```python
from build123d import *

# Parameters (mm, degrees)
SKETCH1_R           = 17
SKETCH1_R_2         = 15
BOSS_EXTRUDE1_DEPTH = 10
BOSS_EXTRUDE2_START = -10
BOSS_EXTRUDE2_DEPTH = 10
CIRPATTERN1_COUNT   = 24


with BuildPart() as part:
    # Sketch1 → Boss-Extrude1 (new body)
    with BuildSketch(Plane.XY):
        Circle(SKETCH1_R)
        Circle(SKETCH1_R_2, mode=Mode.SUBTRACT)
    extrude(amount=BOSS_EXTRUDE1_DEPTH)

    # Sketch2 → Boss-Extrude2 (add)
    with BuildSketch(Plane.XY.offset(10).offset(BOSS_EXTRUDE2_START)):
        with BuildLine():
            ThreePointArc((-2.218945268, 16.854562643), (0, 17.5), (2.218945268, 16.854562643))
            ThreePointArc((2.218945268, 16.854562643), (0, 17), (-2.218945268, 16.854562643))
        make_face()
    boss_extrude2 = extrude(amount=BOSS_EXTRUDE2_DEPTH)

    # CirPattern1: Boss-Extrude2 ×24 about axis
    cirpattern1_axis = Axis((0, 0, 0), (0, 0, 1))
    for i in range(1, CIRPATTERN1_COUNT):
        add(boss_extrude2.rotate(cirpattern1_axis, i * 360 / CIRPATTERN1_COUNT))


solid = part.part
```
Could you check a few things on this model? Use its own coordinates, in mm. Round coordinates to 2 decimals unless told otherwise and drop trailing zeros. Loops run counter-clockwise (first coordinate to the right, second up) from the corner with the lowest first, then second, coordinate; pieces in that order, holes last. Notation, with made-up numbers: (16.25, 78.25) - (68.25, 78.25) arc R26 ccw to (68.25, 104.25) - close; hole circle Ø7 at (19.25, 13.25). An arc over 180 degrees is marked (long way). Answer in a Markdown table with one row per item. Add a question column.
(1) If we section it at A-A (y = 0): Please give me the cut outline in (x, z).
(2) If we mould it in two halves opening along X, with no side actions, what happens to faces 1 (the face through (-4, -15, 10)), 2 (the face through (12.4, -12.35, 4.93)), 3 (the face through (-4.5, -16.91, 4.93))? For each: pulls with the +X half, pulls with the -X half, needs draft (parallel to the pull), parting line crosses it, or undercut.
(3) I need wall thicknesses on line 1 along X through (y, z) = (5.5, 1); line 2 along Y through (x, z) = (6.5, 1.25); line 3 along Y through (x, z) = (2, 6). Which ranges of each line are inside material? Lowest first, please.
(4) If we section it at C-C (z = 1.25): Please give me the cut outline in (x, y), plus the area to 3 significant figures.
(5) I'm going to push flat-ended pins straight in: pin 1 (12 mm diameter, centred on x = 0.5, y = -14, fed in from -Z); pin 2 (4 mm diameter, centred on y = 12, z = 6, fed in from -X); pin 3 (12 mm diameter, centred on x = 3.5, y = -5, fed in from +Z); pin 4 (1.5 mm diameter, centred on y = 13.5, z = 6, fed in from +X). Where does each tip first touch, or does it pass through?
Model answer:
| question | item | result |
|---|---|---|
| 1 | outline | (-17.5, 0) - (-15, 0) - (-15, 10) - (-17.5, 10) - close; (15, 0) - (17.5, 0) - (17.5, 10) - (15, 10) - close |
| 2 | face 1 | needs draft |
| 2 | face 2 | pulls with the +X half |
| 2 | face 3 | undercut |
| 3 | line 1 | x = -16.51 to -13.96, 13.96 to 16.51 |
| 3 | line 2 | y = -15.71 to -13.52, 13.52 to 15.71 |
| 3 | line 3 | y = -16.98 to -14.87, 14.87 to 16.98 |
| 4 | outline | (-16.85, -2.22) arc R4.14 ccw to (-15.71, -6.51) arc R4.14 ccw to (-13.49, -10.35) arc R4.14 ccw to (-10.35, -13.49) arc R4.14 ccw to (-6.51, -15.71) arc R4.14 ccw to (-2.22, -16.85) arc R4.14 ccw to (2.22, -16.85) arc R4.14 ccw to (6.51, -15.71) arc R4.14 ccw to (10.35, -13.49) arc R4.14 ccw to (13.49, -10.35) arc R4.14 ccw to (15.71, -6.51) arc R4.14 ccw to (16.85, -2.22) arc R4.14 ccw to (16.85, 2.22) arc R4.14 ccw to (15.71, 6.51) arc R4.14 ccw to (13.49, 10.35) arc R4.14 ccw to (10.35, 13.49) arc R4.14 ccw to (6.51, 15.71) arc R4.14 ccw to (2.22, 16.85) arc R4.14 ccw to (-2.22, 16.85) arc R4.14 ccw to (-6.51, 15.71) arc R4.14 ccw to (-10.35, 13.49) arc R4.14 ccw to (-13.49, 10.35) arc R4.14 ccw to (-15.71, 6.51) arc R4.14 ccw to (-16.85, 2.22) arc R4.14 ccw to start; hole circle Ø30 at (0, 0) |
| 4 | area | 237 mm² |
| 5 | pin 1 | stops at z = 0 |
| 5 | pin 2 | stops at x = -14.04 |
| 5 | pin 3 | passes through |
| 5 | pin 4 | stops at x = 11.94 |
